```python
from build123d import *

# Parameters (mm, degrees)
SKETCH1_W               = 38.1
SKETCH1_H               = 17.78
BOSS_EXTRUDE1_DEPTH     = 243.84
SKETCH2_W               = 55.88
SKETCH2_H               = 26.67
CUT_EXTRUDE1_DEPTH      = 11.43
SKETCH3_W               = 47.498
SKETCH3_H               = 35.56
CUT_EXTRUDE2_DEPTH      = 10.16
SKETCH4_R               = 1.778
CUT_EXTRUDE3_DEPTH      = 25.4
SKETCH5_R               = 1.016
CUT_EXTRUDE4_DEPTH      = 10.16
SKETCH6_R               = 0.762
CUT_EXTRUDE5_DEPTH      = 6.35
LPATTERN1_COUNT         = 2
LPATTERN1_PITCH         = 38.1
LPATTERN2_COUNT         = 3
LPATTERN2_PITCH         = 12.7
MIRROR2_COPY_1_SKETCH_R = 0.762
MIRROR2_COPY_1_DEPTH    = 6.35
SKETCH7_W               = 5.626456328
SKETCH7_H               = 20.32
CUT_EXTRUDE6_DEPTH      = 248.4382428
MIRROR3_COPY_1_SKETCH_R = 0.762
MIRROR3_COPY_1_DEPTH    = 6.35
MIRROR3_COPY_2_SKETCH_R = 0.762
MIRROR3_COPY_2_DEPTH    = 6.35
MIRROR3_COPY_3_SKETCH_R = 0.762
MIRROR3_COPY_3_DEPTH    = 6.35
SKETCH8_R               = 0.762
BOSS_EXTRUDE2_DEPTH     = 17.78
FILLET1_R               = 10.16
BOSS_EXTRUDE3_DEPTH     = 20.955
SKETCH12_R              = 0.762
CUT_EXTRUDE8_DEPTH      = 248.063150834
FILLET2_R               = 6.35


with BuildPart() as part:
    # Sketch1 → Boss-Extrude1 (new body)
    with BuildSketch(Plane(origin=(0, 0, 0), x_dir=(0, 0, -1), z_dir=(1, 0, 0))):
        with Locations((19.05, -8.89)):
            Rectangle(SKETCH1_W, SKETCH1_H)
    extrude(amount=BOSS_EXTRUDE1_DEPTH)

    # Sketch2 → Cut-Extrude1 (cut)
    with BuildSketch(Plane(origin=(0, 0, 0), x_dir=(1, 0, 0), z_dir=(0, 1, 0))):
        with Locations((157.044117332, 19.05)):
            Rectangle(SKETCH2_W, SKETCH2_H)
    extrude(amount=-CUT_EXTRUDE1_DEPTH, mode=Mode.SUBTRACT)

    # Sketch3 → Cut-Extrude2 (cut)
    with BuildSketch(Plane(origin=(0, 0, 0), x_dir=(1, 0, 0), z_dir=(0, 1, 0))):
        with Locations((99.926945865, 17.78)):
            Rectangle(SKETCH3_W, SKETCH3_H)
    extrude(amount=-CUT_EXTRUDE2_DEPTH, mode=Mode.SUBTRACT)

    # Sketch4 → Cut-Extrude3 (cut)
    with BuildSketch(Plane.XY):
        with Locations((25.4, -8.255)):
            Circle(SKETCH4_R)
        with Locations((203.2, -8.255)):
            Circle(SKETCH4_R)
    extrude(amount=-CUT_EXTRUDE3_DEPTH, mode=Mode.SUBTRACT)

    # Sketch5 → Cut-Extrude4 (cut)
    with BuildSketch(Plane(origin=(0, 0, 0), x_dir=(1, 0, 0), z_dir=(0, 1, 0))):
        with Locations(Location((55.88, 19.05, 0), (0, 0, 270))):
            Circle(SKETCH5_R)
    cut_extrude4 = extrude(amount=-CUT_EXTRUDE4_DEPTH, mode=Mode.SUBTRACT)

    # Sketch6 → Cut-Extrude5 (cut)
    with BuildSketch(Plane(origin=(0, 0, 0), x_dir=(1, 0, 0), z_dir=(0, 1, 0))):
        with Locations(Location((200.66, 29.21, 0), (0, 0, 270))):
            Circle(SKETCH6_R)
        with Locations(Location((200.66, 8.89, 0), (0, 0, 270))):
            Circle(SKETCH6_R)
    cut_extrude5 = extrude(amount=-CUT_EXTRUDE5_DEPTH, mode=Mode.SUBTRACT)

    # LPattern1: Cut-Extrude5 ×2
    with Locations(*[(i * LPATTERN1_PITCH, 0, 0) for i in range(1, LPATTERN1_COUNT)]):
        add(cut_extrude5, mode=Mode.SUBTRACT)

    # LPattern2: Cut-Extrude4 ×3
    with Locations(*[(-i * LPATTERN2_PITCH, 0, 0) for i in range(1, LPATTERN2_COUNT)]):
        add(cut_extrude4, mode=Mode.SUBTRACT)

    # Mirror2: Cut-Extrude5 across plane
    add(cut_extrude5.mirror(Plane.ZX.offset(-8.89)), mode=Mode.SUBTRACT)

    # Mirror2 copy 1 sketch → Mirror2 copy 1 (cut)
    with BuildSketch(Plane(origin=(38.1, -17.78, 0), x_dir=(1, 0, 0), z_dir=(0, -1, 0))):
        with Locations((200.66, -29.21)):
            Circle(MIRROR2_COPY_1_SKETCH_R)
        with Locations((200.66, -8.89)):
            Circle(MIRROR2_COPY_1_SKETCH_R)
    extrude(amount=-MIRROR2_COPY_1_DEPTH, mode=Mode.SUBTRACT)

    # Sketch7 → Cut-Extrude6 (cut, through all)
    with BuildSketch(Plane.XZ.offset(17.78)):
        with Locations((190.226771836, -19.05)):
            Rectangle(SKETCH7_W, SKETCH7_H)
    extrude(amount=-CUT_EXTRUDE6_DEPTH, mode=Mode.SUBTRACT)

    # Mirror3 copy 1 sketch → Mirror3 copy 1 (cut)
    with BuildSketch(Plane(origin=(380.453543672, -17.78, 0), x_dir=(-1, 0, 0), z_dir=(0, -1, 0))):
        with Locations(Location((200.66, 29.21, 0), (0, 0, 270))):
            Circle(MIRROR3_COPY_1_SKETCH_R)
        with Locations(Location((200.66, 8.89, 0), (0, 0, 270))):
            Circle(MIRROR3_COPY_1_SKETCH_R)
    extrude(amount=-MIRROR3_COPY_1_DEPTH, mode=Mode.SUBTRACT)

    # Mirror3 copy 2 sketch → Mirror3 copy 2 (cut)
    with BuildSketch(Plane(origin=(342.353543672, -17.78, 0), x_dir=(-1, 0, 0), z_dir=(0, -1, 0))):
        with Locations(Location((200.66, 29.21, 0), (0, 0, 270))):
            Circle(MIRROR3_COPY_2_SKETCH_R)
        with Locations(Location((200.66, 8.89, 0), (0, 0, 270))):
            Circle(MIRROR3_COPY_2_SKETCH_R)
    extrude(amount=-MIRROR3_COPY_2_DEPTH, mode=Mode.SUBTRACT)

    # Mirror3 copy 3 sketch → Mirror3 copy 3 (cut)
    with BuildSketch(Plane(origin=(380.453543672, 0, 0), x_dir=(-1, 0, 0), z_dir=(0, 1, 0))):
        with Locations((200.66, -29.21)):
            Circle(MIRROR3_COPY_3_SKETCH_R)
        with Locations((200.66, -8.89)):
            Circle(MIRROR3_COPY_3_SKETCH_R)
    extrude(amount=-MIRROR3_COPY_3_DEPTH, mode=Mode.SUBTRACT)

    # Sketch8 → Boss-Extrude2 (add)
    with BuildSketch(Plane.XZ.offset(17.78)):
        with Locations((200.66, -8.89)):
            Circle(SKETCH8_R)
        with Locations((238.76, -8.89)):
            Circle(SKETCH8_R)
        with Locations((238.76, -29.21)):
            Circle(SKETCH8_R)
        with Locations((200.66, -29.21)):
            Circle(SKETCH8_R)
    extrude(amount=-BOSS_EXTRUDE2_DEPTH)

    # Fillet1
    # the kernel refuses this fillet: 10.16 mm, written as the material it takes off along each edge
    with BuildSketch(Plane(origin=(-25.4, -17.78, -38.1), x_dir=(0, 1, 0), z_dir=(1, 0, 0))) as fillet1_piece_1:
        with BuildLine():
            CenterArc((FILLET1_R, FILLET1_R), FILLET1_R, 180, 90)
            Line((0, FILLET1_R), (0, 0))
            Line((0, 0), (FILLET1_R, 0))
        make_face()
    extrude(amount=294.64, mode=Mode.SUBTRACT)

    # Sketch11 → Boss-Extrude3 (add, symmetric)
    with BuildSketch(Plane(origin=(160.743543672, 0, 0), x_dir=(0, 0, -1), z_dir=(1, 0, 0))):
        with BuildLine():
            Line((27.94, -17.78), (38.1, -17.78))
            Line((38.1, -17.78), (38.1, -7.62))
            ThreePointArc((38.1, -7.62), (35.124204897, -14.804204897), (27.94, -17.78))
        make_face()
    extrude(amount=BOSS_EXTRUDE3_DEPTH, both=True)

    # Sketch12 → Cut-Extrude8 (cut, through all)
    with BuildSketch(Plane(origin=(0, -11.43, 0), x_dir=(1, 0, 0), z_dir=(0, 1, 0))):
        with Locations(Location((141.693543672, 29.21, 0), (0, 0, 270))):
            Circle(SKETCH12_R)
        with Locations(Location((179.793543672, 29.21, 0), (0, 0, 270))):
            Circle(SKETCH12_R)
    extrude(amount=-CUT_EXTRUDE8_DEPTH, mode=Mode.SUBTRACT)

    # Fillet2
    fillet2_edges = [part.edges().sort_by_distance(p)[0] for p in [
        (160.743543672, -17.78, -38.1),
    ]]
    fillet(fillet2_edges, radius=FILLET2_R)


solid = part.part
```
The listing builds one solid part. Answer for the finished solid, in the listing's coordinates (mm). A direction names the side the tool comes from. Give positions to 0.01 mm unless a question says otherwise; leave off trailing zeros. Write each loop counter-clockwise with the first axis right and the second up, starting at its lowest first coordinate (ties: lowest second). Pieces come first, ordered by that corner, then holes. Notation, with made-up numbers: (7.5, 69.25) -> (30.5, 69.25) arc R23 cw to (30.5, 83.25) -> close; hole circle Ø9 at (-12, 24.5). An arc over 180 degrees is marked (long way). Write item = value, one per line. Start each with the question number.
1) Which of the six approach directions +Z, -Z, +X, -X, +Y, -Y give full straight-line access (tool end or side, diameter ignored) to faces 1 (the face through (124, -5, -38.1)), 2 (the face through (181.699, -14.9, -35.3)), 3 (the face through (76.178, -5, -18)), 4 (the face through (190, -9, -29.21)), 5 (the face through (157, -6, -5.715))?
2) The part is cut by section D-D, the plane z = -2. Determine the outline of the cut face in (x, y) (3 decimals), and give its area (3 significant figures).
3) Straight lines are drawn through the part: line 1 along X through (y, z) = (-2, -32); line 2 along X through (y, z) = (-1.25, -24); line 3 along X through (y, z) = (-4, -34). For each, find the intervals that lie inside material, in ascending order.
4) The part is cut by section B-B, the plane z = -12.5. Determine the outline of the cut face in (x, y) (3 decimals), and give its area (3 significant figures).
5) The part is cut by section A-A, the plane y = -3. Determine the outline of the cut face in (x, z) (3 decimals).
6) Each of these flat-tipped pins is pushed along its axis until it touches: pin 1 (2 mm diameter, centred on x = 98, z = -9, fed in from +Y); pin 2 (0.9 mm diameter, centred on x = 179.79, z = -8.89, fed in from -Y); pin 3 (13.5 mm diameter, centred on x = 162.5, z = -20.5, fed in from +Y); pin 4 (1.8 mm diameter, centred on x = 204, y = -8.5, fed in from +Z). Where does it stop, or does it pass through?
7) Determine the mould class of faces 6 (the face through (190, -9, -8.89)), 7 (the face through (139.789, -14.9, -35.3)), 8 (the face through (100, -5, -35.56)) for opening direction Z: +Z half, -Z half, draft (parallel to the pull), parting line (faces both ways), or undercut.
8) The part is cut by section C-C, the plane x = 48. Determine the outline of the cut face in (y, z).
Solutions:
q1.face_1 = -Z, +X, -X, +Y, -Y
q1.face_2 = -Z, +X, -Y
q1.face_3 = +Z, +Y
q1.face_4 = +Y, -Y
q1.face_5 = +Y
q2.outline = (0, -17.78) -> (243.84, -17.78) -> (243.84, 0) -> (123.676, 0) -> (123.676, -10.16) -> (76.178, -10.16) -> (76.178, 0) -> (0, 0) -> close; hole circle Ø3.556 at (25.4, -8.255); hole circle Ø3.556 at (203.2, -8.255)
q2.area = 3,830 mm²
q3.line_1 = 0 to 76.18, 123.68 to 129.1, 184.98 to 243.84
q3.line_2 = 0 to 76.18, 123.68 to 129.1, 184.98 to 187.41, 193.04 to 243.84
q3.line_3 = 0 to 76.18, 123.68 to 243.84
q4.outline = (0, -17.78) -> (187.414, -17.78) -> (187.414, 0) -> (184.984, 0) -> (184.984, -11.43) -> (129.104, -11.43) -> (129.104, 0) -> (123.676, 0) -> (123.676, -10.16) -> (76.178, -10.16) -> (76.178, 0) -> (0, 0) -> close; (193.04, -17.78) -> (243.84, -17.78) -> (243.84, 0) -> (193.04, 0) -> close; hole circle Ø3.556 at (25.4, -8.255); hole circle Ø3.556 at (203.2, -8.255)
q4.area = 3,090 mm²
q5.outline = (0, -38.1) -> (243.84, -38.1) -> (243.84, 0) -> (123.676, 0) -> (123.676, -35.56) -> (76.178, -35.56) -> (76.178, 0) -> (0, 0) -> close; hole circle Ø2.032 at (30.48, -19.05); hole circle Ø2.032 at (43.18, -19.05); hole circle Ø2.032 at (55.88, -19.05); hole (129.104, -32.385) -> (184.984, -32.385) -> (184.984, -5.715) -> (129.104, -5.715) -> close; hole (187.414, -29.21) -> (193.04, -29.21) -> (193.04, -8.89) -> (187.414, -8.89) -> close
q6.pin_1 = -10.16
q6.pin_2 = through
q6.pin_3 = -11.43
q6.pin_4 = -25.4
q7.face_6 = undercut
q7.face_7 = draft
q7.face_8 = +Z half
q8.outline = (-17.78, -27.94) arc R10.16 ccw to (-7.62, -38.1) -> (0, -38.1) -> (0, 0) -> (-17.78, 0) -> close
